from build123d import *

# Parameters (mm, degrees)
PAD009_DEPTH    = 2.8
FILLET004_R     = 0.4
POCKET014_DEPTH = 2.801


with BuildPart() as part:
    # Sketch009 (on Face6 of ShapeBinder008) → Pad009 (new body)
    with BuildSketch(Plane.XZ.offset(60.5)):
        with BuildLine():
            Line((37.8, 3.2), (37.8, 0.4))
            Line((37.8, 0.4), (23.8, 0.4))
            ThreePointArc((23.8, 0.4), (23.4, 0), (23.8, -0.4))
            Line((23.8, -0.4), (37.8, -0.4))
            Line((37.8, -0.4), (37.8, -33.8))
            Line((37.8, -33.8), (23.8, -33.8))
            ThreePointArc((23.8, -33.8), (23.4, -34.2), (23.8, -34.6))
            Line((23.8, -34.6), (37.8, -34.6))
            Line((37.8, -34.6), (37.8, -37.4))
            Line((37.8, -37.4), (35.8, -38.15))
            Line((35.8, -38.15), (35.8, -37.4))
            Line((35.8, -37.4), (33, -37.4))
            Line((33, -37.4), (33, -39.4))
            Line((33, -39.4), (25.535898, -37.4))
            Line((25.535898, -37.4), (-25.535898, -37.4))
            Line((-25.535898, -37.4), (-33, -39.4))
            Line((-33, -39.4), (-33, -37.4))
            Line((-33, -37.4), (-35.8, -37.4))
            Line((-35.8, -38.15), (-35.8, -37.4))
            Line((-37.8, -37.4), (-35.8, -38.15))
            Line((-37.8, -37.4), (-37.8, -34.6))
            Line((-37.8, -34.6), (-23.8, -34.6))
            ThreePointArc((-23.8, -34.6), (-23.4, -34.2), (-23.8, -33.8))
            Line((-23.8, -33.8), (-37.8, -33.8))
            Line((-37.8, -33.8), (-37.8, -0.4))
            Line((-37.8, -0.4), (-23.8, -0.4))
            ThreePointArc((-23.8, -0.4), (-23.4, 0), (-23.8, 0.4))
            Line((-23.8, 0.4), (-37.8, 0.4))
            Line((-37.8, 0.4), (-37.8, 3.2))
            Line((-37.8, 3.2), (-35.8, 3.95))
            Line((-35.8, 3.95), (-35.8, 3.2))
            Line((-35.8, 3.2), (-33, 3.2))
            Line((-33, 3.2), (-33, 5.2))
            Line((-33, 5.2), (-25.535898, 3.2))
            Line((-25.535898, 3.2), (25.535898, 3.2))
            Line((25.535898, 3.2), (33, 5.2))
            Line((33, 5.2), (33, 3.2))
            Line((33, 3.2), (35.8, 3.2))
            Line((35.8, 2.45), (35.8, 3.2))
            Line((37.8, 3.2), (35.8, 2.45))
        make_face()
    extrude(amount=-PAD009_DEPTH)

    # Fillet004
    fillet004_edges = [part.edges().sort_by_distance(p)[0] for p in [
        (33, -59.1, 5.2),
        (37.8, -59.1, 3.2),
        (37.8, -59.1, 0.4),
        (37.8, -59.1, -0.4),
        (37.8, -59.1, -33.8),
        (37.8, -59.1, -34.6),
        (37.8, -59.1, -37.4),
        (33, -59.1, -39.4),
        (-37.8, -59.1, -33.8),
        (-37.8, -59.1, -34.6),
        (-37.8, -59.1, -37.4),
        (-33, -59.1, -39.4),
        (-33, -59.1, 5.2),
        (-37.8, -59.1, 3.2),
        (-37.8, -59.1, 0.4),
        (-37.8, -59.1, -0.4),
    ]]
    fillet(fillet004_edges, radius=FILLET004_R)

    # Sketch025 (on Face2 of Fillet004) → Pocket014 (cut, through all)
    with BuildSketch(Plane.XZ.offset(60.5)):
        with BuildLine():
            ThreePointArc((-24, -4.49), (-24.755, -5.245), (-24, -6))
            Line((-24, -6), (-12, -6))
            ThreePointArc((-12, -6), (-11.245, -5.245), (-12, -4.49))
            Line((-24, -4.49), (-12, -4.49))
        make_face()
        with BuildLine():
            ThreePointArc((12, -4.49), (11.245, -5.245), (12, -6))
            Line((12, -6), (24, -6))
            ThreePointArc((24, -6), (24.755, -5.245), (24, -4.49))
            Line((12, -4.49), (24, -4.49))
        make_face()
    extrude(amount=-POCKET014_DEPTH, mode=Mode.SUBTRACT)


solid = part.part
Check sheet for the modelled part. Datum: model origin and axes. Units: mm. A direction names the side the tool comes from. Coordinates: 2 decimals unless noted, no trailing zeros. Loops run counter-clockwise (first coordinate to the right, second up) from the corner with the lowest first, then second, coordinate; pieces in that order, holes last. Notation, with made-up numbers: (-29.5, -15) -> (5.5, -15) arc R15 ccw to (5.5, 0) -> close; hole circle Ø11 at (0.5, 20.25). An arc over 180 degrees is marked (long way). Answer in a Markdown table with one row per item.
1. Material ranges on line 1 along Z through (x, y) = (-35, -59.05); line 2 along Z through (x, y) = (14, -59.6); line 3 along Z through (x, y) = (-30, -58.3), recorded low to high. Write a range as [from, to].
Check values:
| item | result |
|---|---|
| line 1 | z = [-37.4, -34.6], [-33.8, -0.4], [0.4, 3.2] |
| line 2 | z = [-37.4, -6], [-4.49, 3.2] |
| line 3 | z = [-38.6, -34.6], [-33.8, -0.4], [0.4, 4.4] |
2. Sectioned sample at A-A, the plane y = -60. Give the number of separate pieces and of enclosed holes in the cut face, then the cut area to 3 significant figures.
Check values:
| item | result |
|---|---|
| separate pieces | 1 |
| enclosed holes | 2 |
| area | 3,010 mm2 |
3. Sectioned sample at B-B, the plane x = -3.5. Record the boundary of the cut face in (y, z), then the cut area to 3 significant figures.
Check values:
| item | result |
|---|---|
| outline | (-60.5, -37.4) -> (-57.7, -37.4) -> (-57.7, 3.2) -> (-60.5, 3.2) -> close |
| area | 114 mm2 |
4. Release check for a two-part mould opening along Z. For faces 5 (the face through (31, -59, -34.6)), 6 (the face through (36.68, -59.12, -37.82)), 7 (the face through (-37.8, -59, 2)) record: released by +Z, released by -Z, zero draft, split by the parting line, or undercut.
Check values:
| item | result |
|---|---|
| face 5 | undercut |
| face 6 | released by -Z |
| face 7 | zero draft |
5. Go/stop test with flat-tipped pins: pin 1 (0.8 mm diameter, centred on x = -34.5, y = -59.5, fed in from -Z); pin 2 (1.4 mm diameter, centred on x = 34.5, y = -59.5, fed in from +Z); pin 3 (1.4 mm diameter, centred on x = 31.5, y = -58.5, fed in from -Z). Record where each tip stops, or that it passes through.
Check values:
| item | result |
|---|---|
| pin 1 | stops at z = -37.4 |
| pin 2 | stops at z = 3.2 |
| pin 3 | stops at z = -39.19 |
6. Access from +Z, -Z, +X, -X, +Y, -Y to the whole of each face (thin tool, end or side, straight path). Record for faces 1 (the face through (-28.97, -59.12, -38.32)), 2 (the face through (31, -59, -0.4)), 3 (the face through (-34, -59, 3.2)), 4 (the face through (24.755, -59.12, -5.262)).
Check values:
| item | result |
|---|---|
| face 1 | -Z, +Y, -Y |
| face 2 | +X, +Y, -Y |
| face 3 | +Z, +Y, -Y |
| face 4 | +Y, -Y |
